Build history of the part. All positions in model axes, mm. Face numbers are marked on the shaded views. A direction names the side the tool comes from. Round coordinates to 2 decimals unless told otherwise and drop trailing zeros. Write each loop counter-clockwise with the first axis right and the second up, starting at its lowest first coordinate (ties: lowest second). Pieces come first, ordered by that corner, then holes.
1) Saw through at C-C (y = -1.75). Write the cut outline in (x, z), plus the area to 3 significant figures.
2) Saw through at B-B (x = -2). Write the cut outline in (y, z), plus the area to 3 significant figures.
3) Saw through at D-D (z = 0.4). Write the cut outline in (x, y).
4) Which spindle directions (+Z, -Z, +X, -X, +Y, -Y) get a long thin tool onto all of the face, cutting with end or side? Do the marked faces 4 and 5. Say none if no direction does.
5) Saw through at A-A (z = 3.65). Write the cut outline in (x, y).
6) Flat gauge pin, fed straight in: pin 1 (2 mm diameter, centred on y = 2.5, z = 0.5, fed in from +X). Where does the tip first touch, or does it go through?
7) Wall check: probe 1 along X at (y, z) = (0, 3.35); probe 2 along Y at (x, z) = (-1.5, 2.2). Give the ranges that are in metal, low to high.
8) Pull direction Y, two halves, no side cores. Call the marked faces 1, 2 and 3: +Y half, -Y half, draft (parallel to the pull), parting line (faces both ways), or undercut.
from build123d import *

# Parameters (mm, degrees)
SKETCH_W        = 10
SKETCH_H        = 6
PAD_DEPTH       = 3.3
PAD001_DEPTH    = 0.7
SKETCH002_R     = 2.5
POCKET_DEPTH    = 5
POCKET001_DEPTH = 6
FILLET_R        = 0.2


with BuildPart() as part:
    # Sketch → Pad (new body)
    with BuildSketch(Plane.XY):
        Rectangle(SKETCH_W, SKETCH_H)
    extrude(amount=PAD_DEPTH)

    # Sketch001 (on Face6 of Pad) → Pad001 (join)
    with BuildSketch(Plane.XY.offset(3.3)):
        with BuildLine():
            Line((0, 3), (3, 3))
            Line((3, 3), (3, 0))
            ThreePointArc((0, -3), (2.12132, -2.12132), (3, 0))
            Line((0, -3), (-3, -3))
            Line((-3, -3), (-3, -2e-06))
            ThreePointArc((0, 3), (-2.121321, 2.12132), (-3, -2e-06))
        make_face()
    extrude(amount=PAD001_DEPTH)

    # Sketch002 (on Face12 of Pad001) → Pocket (cut)
    with BuildSketch(Plane.XY.offset(4)):
        Circle(SKETCH002_R)
    extrude(amount=-POCKET_DEPTH, mode=Mode.SUBTRACT)

    # Sketch003 (on Face8 of Pocket) → Pocket001 (cut)
    with BuildSketch(Plane.XZ.offset(3)):
        Polygon((-2.4, 0), (2.4, 0), (5, 2.6), (7.104516, 2.6), (7.104516, -2.6), (-7.104516, -2.6), (-7.104516, 2.6), (-5, 2.6), align=None)
    extrude(amount=-POCKET001_DEPTH, mode=Mode.SUBTRACT)

    # Fillet
    fillet_edges = [part.edges().sort_by_distance(p)[0] for p in [
        (-5, 0, 3.3),
        (5, 0, 3.3),
    ]]
    fillet(fillet_edges, radius=FILLET_R)


solid = part.part
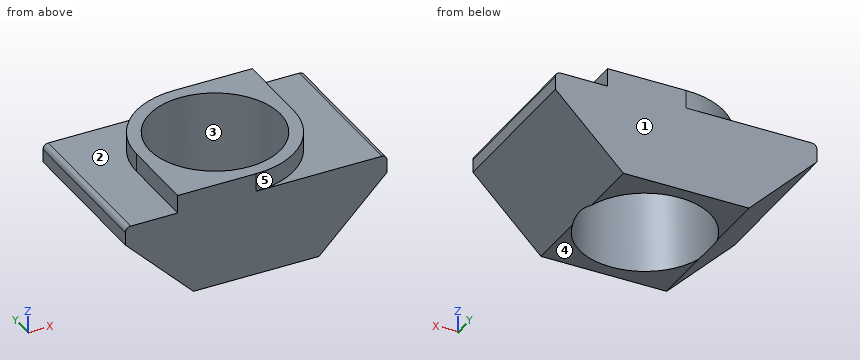
Evaluation:
1. outline: (-5, 2.6) - (-2.4, 0) - (-1.79, 0) - (-1.79, 4) - (-3, 4) - (-3, 3.3) - (-4.8, 3.3) arc R0.2 ccw to (-5, 3.1) - close; (1.79, 0) - (2.4, 0) - (5, 2.6) - (5, 3.1) arc R0.2 ccw to (4.8, 3.3) - (2.44, 3.3) - (2.44, 4) - (1.79, 4) - close
1. area: 15.7 mm2
2. outline: (-3, 0) - (-1.5, 0) - (-1.5, 4) - (-3, 4) - close; (1.5, 0) - (3, 0) - (3, 3.3) - (2.24, 3.3) - (2.24, 4) - (1.5, 4) - close
2. area: 11.5 mm2
3. outline: (-2.8, -3) - (2.8, -3) - (2.8, 3) - (-2.8, 3) - close; hole circle Ø5 at (0, 0)
4. face 4: -Z, +X, -X, +Y, -Y
4. face 5: +Z, +X, -Y
5. outline: (-3, -3) - (0, -3) arc R3 ccw to (3, 0) - (3, 3) - (0, 3) arc R3 ccw to (-3, 0) - close; hole circle Ø5 at (0, 0)
6. pin 1: stops at x = 3.9
7. probe 1: x = -3 to -2.5, 2.5 to 3
7. probe 2: y = -3 to -2, 2 to 3
8. face 1: +Y half
8. face 2: draft
8. face 3: undercut
